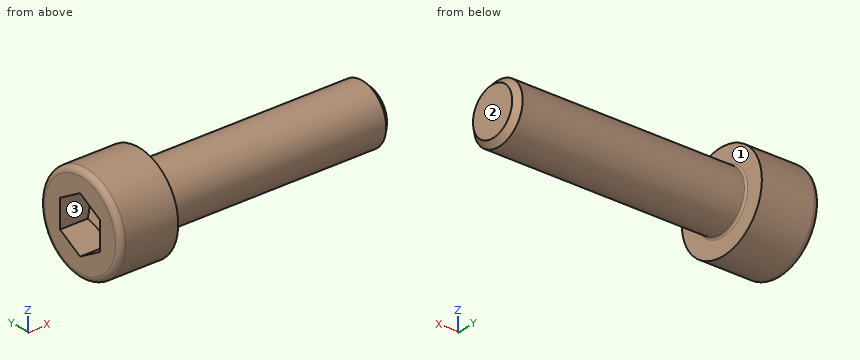
Autodesk Inventor part; units mm, degrees
ref_plane "Work Plane1" through (29, 0, 0) normal (0, -1, 0) x (1, 0, 0)
ref_plane "YZ Plane" through (0, 0, 0) normal (1, 0, 0) x (0, 1, 0)
ref_plane "XZ Plane" through (0, 0, 0) normal (0, 1, 0) x (-1, 0, 0)
sketch "Sketch1" plane through (0, 0, 0) normal (0, 0, 1) x (1, 0, 0)
  line L0 (-1.2192, 0) -> (19.05, 0)
  line L1 (19.05, 0) -> (19.05, 2.413)
  line L2 (19.05, 2.413) -> (1.191, 2.413)
  line L3 (1.191, 2.413) -> (0.0001, 2.413)
  line L4 (0.0001, 2.413) -> (0, 2.413)
  line L5 (0, 2.413) -> (0, 3.9624)
  line L6 (0, 3.9624) -> (-4.826, 3.9624)
  line L7 (-4.826, 3.9624) -> (-4.826, 2.2877)
  line L8 (-4.826, 2.2877) -> (-2.54, 2.2877)
  line L9 (-2.54, 2.2877) -> (-1.2192, 0)
  line L10 (-9.6012, 0) -> (23.8252, 0)
  line L11 (0, -0.7925) -> (0, 4.7549)
  line L12 (1.191, 2.413) -> (0, 2.413) construction
  dimension "d1" = 17.859
  dimension "d2" = 1.1908
  dimension "d3" = 4.826
  dimension "d4" = 2.286
  dimension "d5" = 60
  dimension "d6" = 4.826
  dimension "d7" = 4.826
  dimension "d8" = 4.5754
  dimension "d9" = 7.9248
  dimension "d26" = 19.05
revolve "Body" add sketch "Sketch1" angle 360 about axis through (-1.2192, 0, 0) along (1, 0, 0)
sketch "Sketch2" plane through (-4.826, 0, 0) normal (-1, 0, 0) x (0, 0, 1)
  circle A0 centre (0, 0) radius 2.2877
  line L0 (0, -5.5474) -> (0, 5.5474)
  line L1 (-5.5474, 0) -> (5.5474, 0)
  line L2 (2.2877, 0) -> (1.1438, -1.9812)
  line L3 (1.1438, -1.9812) -> (-1.1438, -1.9812)
  line L4 (-1.1438, -1.9812) -> (-2.2877, 0)
  line L5 (-2.2877, 0) -> (-1.1438, 1.9812)
  line L6 (-1.1438, 1.9812) -> (1.1438, 1.9812)
  line L7 (1.1438, 1.9812) -> (2.2877, 0)
extrude "Slot" add sketch "Sketch2" against normal up to next contours L7 A0 | A0 L2 | L6 L0 A0 | A0 L0 L3 | L0 L6 A0 | A0 L3 L0 | L4 A0 | A0 L5
fillet "Fillet1" radius 0.4572 1 edges at (-4.826, -3.9624, 0)
thread "Thread"
chamfer "Chamfer1" distance 0.4724 distance2 0.4724 1 edges at (19.05, -2.413, 0) measured on face at (19.05, -1.2173, -0.6389)
ref_plane "Work Plane1" through (29, 0, 0) normal (0, -1, 0) x (1, 0, 0)
fillet "Fillet2" radius 0.1524 1 edges at (0.0001, -2.413, 0)
equation "\"d1\" = GEL"
equation "\"d3\" = KOH"
equation "\"d4\" = INTI"
equation "\"d6\" = GD"
equation "\"d7\" = BDM"
equation "\"d8\" = 1.1547 * SW"
equation "\"d9\" = KOD"
equation "\"d26\" = NLG"
equation "\"d30\" = R"
equation "\"d17\" = RR"
equation "\"d13\" = GEL"
equation "\"d15\" = -0.5 * SPD + 0.5 * GD"
equation "\"d16\" = GUL"
equation "\"GD\" = 4.826"
equation "\"NLG\" = 19.05"
equation "\"GEL\" = 17.85905"
equation "\"KOD\" = 7.9248"
equation "\"KOH\" = 4.826"
equation "\"INTI\" = 2.286"
equation "\"GAL\" = 1.19075"
equation "\"GUL\" = 0.47244"
equation "\"BDM\" = 4.826"
equation "\"SW\" = 3.9624"
equation "\"RR\" = 0.4572"
equation "\"SPD\" = 3.88112"
equation "\"R\" = 0.1524"
equation "\"PHH\" = 0.127"
equation "\"GD1\" = SPD"
equation "\"THREADDIA\" = 4.826"
equation "\"FAWI\" = 45deg"
equation "\"KOH1\" = 4.3434"
equation "\"NND\" = 4.826"
equation "\"TOA\" = 30deg"
equation "\"E0\" = 1.155 * SW"
properties part number "am-1047" material "Steel, Mild"
Read the model definition and answer for the solid it produces. Units are mm, in the model's axes. Face numbers are marked on the shaded views. A direction names the side the tool comes from. Coordinates: 2 decimals unless noted, no trailing zeros. Loops run counter-clockwise (first coordinate to the right, second up) from the corner with the lowest first, then second, coordinate; pieces in that order, holes last. Notation, with made-up numbers: (64.25, 64.5) -> (119.25, 64.5) arc R3 ccw to (119.25, 69.5) -> close; hole circle Ø9 at (88.25, 38.25). An arc over 180 degrees is marked (long way). Answer in a Markdown table with one row per item.
Item 1: A cutting plane is placed at B-B on x = 14.75. Determine the outline of the cut face in (y, z), plus the area to 3 significant figures.
Returned:
| item | result |
|---|---|
| outline | circle Ø4.83 at (0, 0) |
| area | 18.3 mm^2 |
Item 2: Each of these flat-tipped pins is pushed along its axis until it touches: P1, Ø4, axis at x = 3.5, y = -0.5, coming from the +Z side; P2, Ø2, axis at x = 6.5, z = -1, coming from the +Y side. Where does it stop, or does it pass through?
Returned:
| item | result |
|---|---|
| P1 | stops at z = 2.41 |
| P2 | stops at y = 2.41 |
Item 3: For the marked faces 1, 2 and 3, determine the directions among +Z, -Z, +X, -X, +Y, -Y from which every point of the face is accessible in a straight line to the end or side of a thin tool.
Returned:
| item | result |
|---|---|
| face 1 | +X |
| face 2 | +Z, -Z, +X, +Y, -Y |
| face 3 | -X |
Item 4: Straight lines are drawn through the part: line 1 along Y through (x, z) = (12, 0.75); line 2 along X through (y, z) = (-2.75, 1.75); line 3 along Z through (x, y) = (9.25, -1.25). For each, find the intervals that lie inside material, in ascending order. Write a range as [from, to].
Returned:
| item | result |
|---|---|
| line 1 | y = [-2.29, 2.29] |
| line 2 | x = [-4.83, 0] |
| line 3 | z = [-2.06, 2.06] |
Item 5: A cutting plane is placed at A-A on x = -3. Determine the outline of the cut face in (y, z), plus the area to 3 significant figures.
Returned:
| item | result |
|---|---|
| outline | circle Ø7.92 at (0, 0); hole (-1.98, -1.14) -> (0, -2.29) -> (1.98, -1.14) -> (1.98, 1.14) -> (0, 2.29) -> (-1.98, 1.14) -> close |
| area | 35.7 mm^2 |
